Could you check a few things on this model? Use its own coordinates, in mm. Face numbers are marked on the shaded views. A direction names the side the tool comes from. Round coordinates to 2 decimals unless told otherwise and drop trailing zeros. Answer in a Markdown table with one row per item.
from build123d import *

# Parameters (mm, degrees)
F0_W        = 30
F0_H        = 30
F1_DEPTH    = 25
F2_R        = 7.25
F3_DEPTH    = 25
F4_SIZE2    = 24.99999
F4_SIZE     = 4.99999
F5_T1_DEPTH = 102.9607936575
F5_T3_DEPTH = 102.9607936575
F5_T5_DEPTH = 102.9607936575
F5_T7_DEPTH = 102.9607936575
F7_DEPTH    = 25
F8_R        = 11
F9_DEPTH    = 4


# Not quite as in the source:
# - a fillet or chamfer that OpenCascade refuses, or shapes differently, is made with other operations: its cross-section is extruded or revolved along the edge and cut away or added
# - a fillet or chamfer is up to 0.001 mm smaller than in the source, because OpenCascade refuses the exact size


with BuildPart() as f1:
    # F0 (on Top) → F1 (new body)
    with BuildSketch(Plane.XY):
        Rectangle(F0_W, F0_H)
    extrude(amount=F1_DEPTH)

    # F2 (on face) → F3 (cut)
    with BuildSketch(Plane.XY.offset(25)):
        Circle(F2_R)
    extrude(amount=-F3_DEPTH, mode=Mode.SUBTRACT)

    # F4 (size 5 and 25 in the source; OpenCascade refuses exactly that, so slightly less here)
    f4_edges = [f1.edges().sort_by_distance(p)[0] for p in [
        (15, 0, 25),
        (0, 15, 25),
        (-15, 0, 25),
        (0, -15, 25),
    ]]
    f4_side = f1.faces().sort_by_distance((14.575736, 0, 25))[0]
    chamfer(f4_edges, length=F4_SIZE, length2=F4_SIZE2, reference=f4_side)

    # F5: fillet of radius 8 on 4 edges, made by hand

    # F5_s2 → F5_t1 (cut)
    with BuildSketch(Plane(origin=(-7.5925826886, 7.5925826886, 37.9629741838), x_dir=(0.7071067812, 0.7071067812, 0), z_dir=(0.1924498046, -0.1924498046, -0.9622505627))):
        with BuildLine():
            ThreePointArc((5.5470023036, 15.0748135762), (0, 17.3102003677), (-5.5470023036, 15.0748135762))
            Line((-5.5470023036, 15.0748135762), (0, 20.4124196641))
            Line((0, 20.4124196641), (5.5470023036, 15.0748135762))
        make_face()
    extrude(amount=F5_T1_DEPTH, mode=Mode.SUBTRACT)

    # F5_s4 → F5_t3 (cut)
    with BuildSketch(Plane(origin=(-7.5925826886, -7.5925826886, 37.9629741838), x_dir=(-0.7071067812, 0.7071067812, 0), z_dir=(0.1924498046, 0.1924498046, -0.9622505627))):
        with BuildLine():
            ThreePointArc((-5.5470023036, 15.0748135762), (0, 17.3102003677), (5.5470023036, 15.0748135762))
            Line((5.5470023036, 15.0748135762), (0, 20.4124196641))
            Line((0, 20.4124196641), (-5.5470023036, 15.0748135762))
        make_face()
    extrude(amount=F5_T3_DEPTH, mode=Mode.SUBTRACT)

    # F5_s6 → F5_t5 (cut)
    with BuildSketch(Plane(origin=(7.5925826886, -7.5925826886, 37.9629741838), x_dir=(-0.7071067812, -0.7071067812, 0), z_dir=(-0.1924498046, 0.1924498046, -0.9622505627))):
        with BuildLine():
            ThreePointArc((-5.5470023036, 15.0748135762), (0, 17.3102003677), (5.5470023036, 15.0748135762))
            Line((5.5470023036, 15.0748135762), (0, 20.4124196641))
            Line((0, 20.4124196641), (-5.5470023036, 15.0748135762))
        make_face()
    extrude(amount=F5_T5_DEPTH, mode=Mode.SUBTRACT)

    # F5_s8 → F5_t7 (cut)
    with BuildSketch(Plane(origin=(7.5925826886, 7.5925826886, 37.9629741838), x_dir=(0.7071067812, -0.7071067812, 0), z_dir=(-0.1924498046, -0.1924498046, -0.9622505627))):
        with BuildLine():
            ThreePointArc((5.5470023036, 15.0748135762), (0, 17.3102003677), (-5.5470023036, 15.0748135762))
            Line((-5.5470023036, 15.0748135762), (0, 20.4124196641))
            Line((0, 20.4124196641), (5.5470023036, 15.0748135762))
        make_face()
    extrude(amount=F5_T7_DEPTH, mode=Mode.SUBTRACT)

    # F6 (on face) → F7 (cut)
    with BuildSketch(Plane(origin=(0, 0, 0), x_dir=(1, 0, 0), z_dir=(0, 0, -1))):
        with BuildLine():
            ThreePointArc((0, 15), (10.6066017178, 10.6066017178), (15, 0))
            Line((15, 0), (15, 7.1610644072))
            add(Edge.make_bspline(
                [(7.1610644072, 15), (14.9945107468, 14.9945107468), (15, 7.1610644072)],
                knots=[2.3761301528, 2.3761301528, 2.3761301528, 3.9070551544, 3.9070551544, 3.9070551544], degree=2, weights=[1, 0.7210619814, 1]))
            Line((7.1610644072, 15), (0, 15))
        make_face()
        with BuildLine():
            ThreePointArc((-15, 0), (-10.6066017178, 10.6066017178), (0, 15))
            Line((0, 15), (-7.1610644072, 15))
            add(Edge.make_bspline(
                [(-15, 7.1610644072), (-14.9945107468, 14.9945107468), (-7.1610644072, 15)],
                knots=[2.3761301528, 2.3761301528, 2.3761301528, 3.9070551544, 3.9070551544, 3.9070551544], degree=2, weights=[1, 0.7210619814, 1]))
            Line((-15, 7.1610644072), (-15, 0))
        make_face()
        with BuildLine():
            Line((-7.1610644072, -15), (0, -15))
            ThreePointArc((0, -15), (-10.6066017178, -10.6066017178), (-15, 0))
            Line((-15, 0), (-15, -7.1610644072))
            add(Edge.make_bspline(
                [(-7.1610644072, -15), (-14.9945107468, -14.9945107468), (-15, -7.1610644072)],
                knots=[2.3761301528, 2.3761301528, 2.3761301528, 3.9070551544, 3.9070551544, 3.9070551544], degree=2, weights=[1, 0.7210619814, 1]))
        make_face()
        with BuildLine():
            Line((15, -7.1610644072), (15, 0))
            ThreePointArc((15, 0), (10.6066017178, -10.6066017178), (0, -15))
            Line((0, -15), (7.1610644072, -15))
            add(Edge.make_bspline(
                [(15, -7.1610644072), (14.9945107468, -14.9945107468), (7.1610644072, -15)],
                knots=[2.3761301528, 2.3761301528, 2.3761301528, 3.9070551544, 3.9070551544, 3.9070551544], degree=2, weights=[1, 0.7210619814, 1]))
        make_face()
    extrude(amount=-F7_DEPTH, mode=Mode.SUBTRACT)

    # F8 (on face) → F9 (cut)
    with BuildSketch(Plane(origin=(0, 0, 0), x_dir=(1, 0, 0), z_dir=(0, 0, -1))):
        Circle(F8_R)
    extrude(amount=-F9_DEPTH, mode=Mode.SUBTRACT)


solid = f1.part
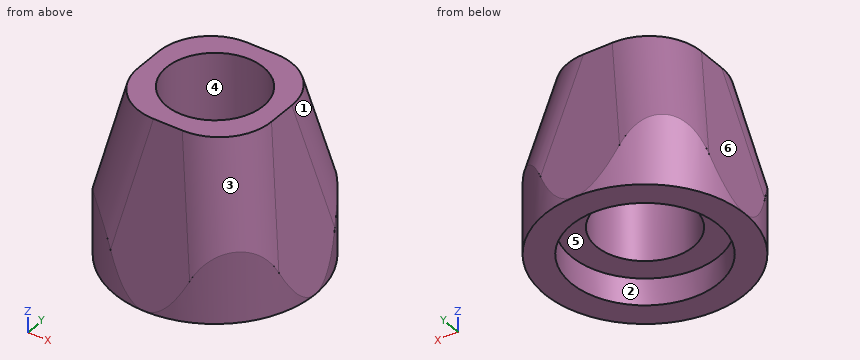
1) Please list where these lines run through material, in increasing order: line 1 (X direction, y = 0, z = 1.95); line 2 (X direction, y = -3.5, z = 8.75); line 3 (Y direction, x = -4, z = 18.5).
Findings:
| item | result |
|---|---|
| line 1 | x = -14.61 to -11, 11 to 14.61 |
| line 2 | x = -13.25 to -6.35, 6.35 to 13.25 |
| line 3 | y = -11.28 to -6.05, 6.05 to 11.28 |
2) For the marked faces 1 and 2, which set-ups out of +Z, -Z, +X, -X, +Y, -Y let a thin tool reach every point of the face, with its end or its side?
Findings:
| item | result |
|---|---|
| face 1 | +Z, +X, +Y |
| face 2 | -Z |
3) For pin 1 (6 mm diameter, centred on y = 5, z = 13, fed in from -X); pin 2 (2 mm diameter, centred on y = -9, z = 9.5, fed in from +X); pin 3 (3 mm diameter, centred on x = -2.5, z = 15, fed in from +Y); pin 4 (2 mm diameter, centred on x = -6, y = 1.5, fed in from +Z), each with a flat end and sliding along its axis, tell me the tip position at first contact or that it passes through.
Findings:
| item | result |
|---|---|
| pin 1 | stops at x = -13 |
| pin 2 | stops at x = 12.67 |
| pin 3 | stops at y = 12.3 |
| pin 4 | passes through |
4) Thinking about a two-plate mould opening in X: for the marked faces 3, 4, 5 and 6, which applies, +X half, -X half, draft (parallel to the pull), parting line (faces both ways), or undercut?
Findings:
| item | result |
|---|---|
| face 3 | +X half |
| face 4 | undercut |
| face 5 | undercut |
| face 6 | -X half |
